Part model, mm, in its own coordinate system. Give positions to 0.01 mm unless a question says otherwise; leave off trailing zeros. Write each loop counter-clockwise with the first axis right and the second up, starting at its lowest first coordinate (ties: lowest second). Pieces come first, ordered by that corner, then holes. Notation, with made-up numbers: M 84.25,47.5 L 95.25,47.5 A32 cw 95.25,85.5 Z; hole C 70.5,-39 d8. An arc over 180 degrees is marked long. Answer as CSV lines item,"result". Start each with the question number.
Item 1: Wall check: L1, parallel to X at y = 718, z = 3.35; L2, parallel to Y at x = -87, z = 0.9; L3, parallel to Y at x = -42.5, z = 2.4. Give the ranges that are in metal, low to high. Write a range as from..to.
Item 2: Band-saw the part on D-D, the plane x = -127. List the corners of the cut face in (y, z).
Item 3: Band-saw the part on C-C, the plane x = 92.5. List the corners of the cut face in (y, z), then the cut area to 3 significant figures.
Item 4: Band-saw the part on A-A, the plane y = 670. List the corners of the cut face in (x, z).
from build123d import *

# Parameters (mm, degrees)
F0_W     = 457.2
F0_H     = 914.4
F1_DEPTH = 4.7752
F2_R     = 228.59999
F3_W     = 203.2
F3_H     = 203.2
F4_DEPTH = 25.399999693


# Not quite as in the source:
# - a fillet or chamfer is up to 0.001 mm smaller than in the source, because OpenCascade refuses the exact size
# - ends of sketch curves that miss each other by under 0.0002 mm in the source are joined


with BuildPart() as f1:
    # F0 (on Top) → F1 (new body)
    with BuildSketch(Plane.XY):
        with Locations((0, 457.2)):
            Rectangle(F0_W, F0_H)
    extrude(amount=F1_DEPTH)

    # F2 (radius 228.6 in the source; OpenCascade refuses exactly that, so slightly less here)
    f2_edges = [f1.edges().sort_by_distance(p)[0] for p in [
        (228.6, 0, 2.3876),
        (-228.6, 0, 2.3876),
    ]]
    fillet(f2_edges, radius=F2_R)

    # F3 (on face) → F4 (intersect)
    with BuildSketch(Plane.XY.offset(4.7752)):
        with BuildLine():
            Line((-228.6, 914.4), (-228.6, 228.59999))
            ThreePointArc((-228.6, 228.59999), (-161.6446131082, 66.9553868918), (-1e-05, 0))
            ThreePointArc((-1e-05, 0), (161.6446131082, 66.9553868918), (228.6, 228.59999))
            Line((228.6, 228.59999), (228.6, 914.4))
            Line((228.6, 914.4), (-228.6, 914.4))
        make_face()
        with Locations((0, 660.4)):
            Rectangle(F3_W, F3_H, mode=Mode.SUBTRACT)
    extrude(amount=-F4_DEPTH, mode=Mode.INTERSECT)


solid = f1.part
Output:
1,L1,"-228.6..-101.6, 101.6..228.6"
1,L2,"17.2..558.8, 762..914.4"
1,L3,"3.99..558.8, 762..914.4"
2,outline,"M 38.52,0 L 914.4,0 L 914.4,4.78 L 38.52,4.78 Z"
3,outline,"M 19.55,0 L 558.8,0 L 558.8,4.78 L 19.55,4.78 Z; M 762,0 L 914.4,0 L 914.4,4.78 L 762,4.78 Z"
3,area,"3,300 mm²"
4,outline,"M -228.6,0 L -101.6,0 L -101.6,4.78 L -228.6,4.78 Z; M 101.6,0 L 228.6,0 L 228.6,4.78 L 101.6,4.78 Z"
